Design review of the part built by this model. Coordinates are the model's own, in mm. A direction names the side the tool comes from. Coordinates: 2 decimals unless noted, no trailing zeros. Loops run counter-clockwise (first coordinate to the right, second up) from the corner with the lowest first, then second, coordinate; pieces in that order, holes last. Notation, with made-up numbers: (24.25, 11) -> (29.25, 11) arc R20 cw to (29.25, 15) -> close; hole circle Ø8 at (-26, 34). An arc over 180 degrees is marked (long way). Answer as a JSON object with one key per item and string values.
```python
from build123d import *

# Parameters (mm, degrees)
SKETCH_1_R      = 1.65
EXTRUDE_1_DEPTH = 3
FILLET_1_R      = 20


with BuildPart() as part:
    # 草图1 → 凸台-拉伸1 (new body)
    with BuildSketch(Plane.XY):
        Polygon((-81.159641577, 128.097043492), (-81.160013188, 69.97789137), (-33.727366855, 19.978035289), (-81.160652583, -30.022108629), (-81.161024198, -88.141807947), (-6.159655428, -9.081730725), (68.841408465, -88.142097171), (68.841260976, -30.022397853), (21.408168061, 19.97792898), (68.841007207, 69.977602148), (68.840859718, 128.096754271), (-6.159543366, 49.037694994), align=None)
        with Locations((-71.160908341, -70.022108629)):
            Circle(SKETCH_1_R, mode=Mode.SUBTRACT)
        with Locations((-71.160780462, -50.022108629)):
            Circle(SKETCH_1_R, mode=Mode.SUBTRACT)
        with Locations((-71.160652583, -30.022108629)):
            Circle(SKETCH_1_R, mode=Mode.SUBTRACT)
        with Locations((58.841362483, -70.02235929)):
            Circle(SKETCH_1_R, mode=Mode.SUBTRACT)
        with Locations((58.841311729, -50.02235929)):
            Circle(SKETCH_1_R, mode=Mode.SUBTRACT)
        with Locations((58.841260976, -30.02235929)):
            Circle(SKETCH_1_R, mode=Mode.SUBTRACT)
        with Locations((-71.160013188, 69.97787102)):
            Circle(SKETCH_1_R, mode=Mode.SUBTRACT)
        with Locations((-71.159885309, 89.977871019)):
            Circle(SKETCH_1_R, mode=Mode.SUBTRACT)
        with Locations((-71.15975743, 109.977871019)):
            Circle(SKETCH_1_R, mode=Mode.SUBTRACT)
        with Locations((58.841007207, 69.977620361)):
            Circle(SKETCH_1_R, mode=Mode.SUBTRACT)
        with Locations((58.840956453, 89.977620361)):
            Circle(SKETCH_1_R, mode=Mode.SUBTRACT)
        with Locations((58.840905699, 109.977620361)):
            Circle(SKETCH_1_R, mode=Mode.SUBTRACT)
    extrude(amount=EXTRUDE_1_DEPTH)

    # 圆角1
    fillet_1_edges = [part.edges().sort_by_distance(p)[0] for p in [
        (21.408168061, 19.97792898, 1.5),
        (-6.159655428, -9.081730725, 1.5),
        (-33.727366855, 19.978035289, 1.5),
        (-6.159543366, 49.037694994, 1.5),
    ]]
    fillet(fillet_1_edges, radius=FILLET_1_R)


solid = part.part
```
1) Add section C-C, the plane z = 2.25. Count the separate pieces of the cut face and the enclosed holes in it, and give its area (3 significant figures).
Completed:
{"separate pieces": "1", "enclosed holes": "12", "area": "16,100 mm²"}
2) Add section A-A, the plane y = -60.5. Give the boundary of the cut face in (x, z).
Completed:
{"outline": "(-81.16, 0) -> (-54.94, 0) -> (-54.94, 3) -> (-81.16, 3) -> close; (42.62, 0) -> (68.84, 0) -> (68.84, 3) -> (42.62, 3) -> close"}
3) Add section B-B, the plane x = -57. Give the boundary of the cut face in (y, z), and give its area (3 significant figures).
Completed:
{"outline": "(-62.67, 0) -> (-4.55, 0) -> (-4.55, 3) -> (-62.67, 3) -> close; (44.51, 0) -> (102.63, 0) -> (102.63, 3) -> (44.51, 3) -> close", "area": "349 mm²"}
4) For faces 1 (the flat face through (51.894, -12.158, 1.479)), 2 (the flat face through (-50.49, 95.77, 1.48)), 3 (the flat face through (-63.73, -11.65, 1.48)), list the 3-axis set-ups (+Z, -Z, +X, -X, +Y, -Y) from which the entire face can be reached by the end or side of a thin tool; tool diameter is ignored.
Completed:
{"face 1": "+Z, -Z, +X", "face 2": "+Z, -Z, +Y", "face 3": "+Z, -Z, -X"}
5) Wall thickness on probe 1 along X at (y, z) = (-22.5, 0.85); probe 2 along Y at (x, z) = (-54.5, 1.9); probe 3 along Y at (x, z) = (-49, 0.75): over which ranges is each line inside the solid? List them lowest first.
Completed:
{"probe 1": "-74.02 to -18.62, 6.3 to 61.71", "probe 2": "-60.04 to -1.92, 41.87 to 99.99", "probe 3": "-54.24 to 3.88, 36.08 to 94.2"}
6) The part is to be moulded in two halves that separate along Y. For faces 4 (the cylindrical face through (-6.4, 58.1, 1.5)), 5 (the flat face through (-7, 21, 3)), 6 (the cylindrical face through (28.977, 20.19, 1.521)), say which applies: pulls with the +Y half, pulls with the -Y half, needs draft (parallel to the pull), parting line crosses it, or undercut.
Completed:
{"face 4": "pulls with the +Y half", "face 5": "needs draft", "face 6": "undercut"}
7) Add section D-D, the plane x = 0. Give the boundary of the cut face in (y, z), and give its area (3 significant figures).
Completed:
{"outline": "(-19.11, 0) -> (59.07, 0) -> (59.07, 3) -> (-19.11, 3) -> close", "area": "235 mm²"}
